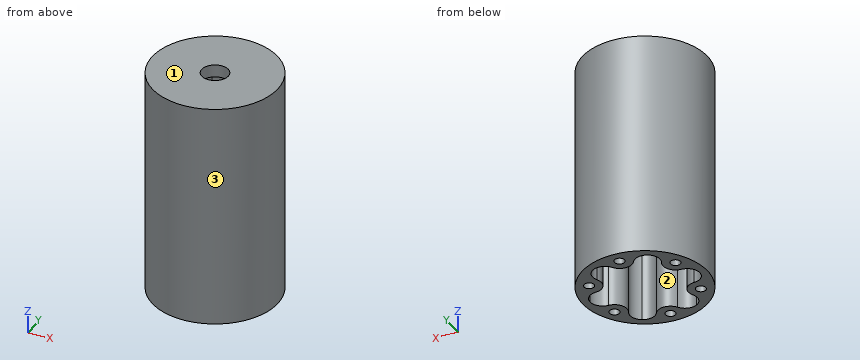
Autodesk Inventor part; units mm, degrees
ref_plane "YZ Plane" through (0, 0, 0) normal (1, 0, 0) x (0, 1, 0)
ref_plane "XZ Plane" through (0, 0, 0) normal (0, 1, 0) x (-1, 0, 0)
ref_plane "XY Plane" through (0, 0, 0) normal (0, 0, 1) x (1, 0, 0)
sketch "Sketch1" plane through (0, 0, 0) normal (0, 0, 1) x (1, 0, 0)
  circle A0 centre (0, 0) radius 15.875
  circle A1 centre (0, 0) radius 13.97
  dimension "d0" = 31.75
  dimension "d1" = 27.94
extrude "Extrusion1" add sketch "Sketch1" along normal blind 57.15
sketch "Sketch2" plane through (0, 0, 0) normal (0, 0, -1) x (-1, 0, 0)
  line L0 (0, 0) -> (0, 12.7)
  circle A0 centre (0, 12.7) radius 1.27
  circle A1 centre (0, 12.7) radius 3.175
  circle A2 centre (-10.9985, 6.35) radius 3.175
  circle A3 centre (-10.9985, 6.35) radius 1.27
  circle A4 centre (-10.9985, -6.35) radius 3.175
  circle A5 centre (-10.9985, -6.35) radius 1.27
  circle A6 centre (0, -12.7) radius 3.175
  circle A7 centre (0, -12.7) radius 1.27
  circle A8 centre (10.9985, -6.35) radius 3.175
  circle A9 centre (10.9985, -6.35) radius 1.27
  circle A10 centre (10.9985, 6.35) radius 3.175
  circle A11 centre (10.9985, 6.35) radius 1.27
  dimension "d4" = 12.7
  dimension "d5" = 2.54
  dimension "d6" = 6.35
  dimension "d9" = 360
extrude "Extrusion2" add sketch "Sketch2" against normal up to surface (57.15 mm away) contours A0 | A1 | A2 | A3 | A4 | A5 | A6 | A7 | A8 | A9 | A10 | A11
extrude "Extrusion3" cut sketch "Sketch2" against normal blind 12.7 contours A0 | A3 | A5 | A7 | A9 | A11
sketch "Sketch3" plane through (0, 0, 57.15) normal (0, 0, 1) x (1, 0, 0)
  circle A0 centre (0, 0) radius 3.3655
  circle A1 centre (0, 0) radius 13.97
  dimension "d15" = 6.731
extrude "Extrusion4" add sketch "Sketch3" against normal blind 3.175
fillet "Fillet1" radius 3.175 12 edges at (-3.0337, 13.6366, 26.9875) (3.0337, 13.6366, 26.9875) (13.3265, 4.191, 26.9875) (10.2928, 9.4456, 26.9875) (13.3265, -4.191, 26.9875) (10.2928, -9.4456, 26.9875) (3.0337, -13.6366, 26.9875) (-3.0337, -13.6366, 26.9875) (-10.2928, -9.4456, 26.9875) (-13.3265, -4.191, 26.9875) (-13.3265, 4.191, 26.9875) (-10.2928, 9.4456, 26.9875)
properties part number "FixedCylinderWireStorage" material "ABS Plastic"
Could you check a few things on this model? Use its own coordinates, in mm. Face numbers are marked on the shaded views. Round coordinates to 2 decimals unless told otherwise and drop trailing zeros. Put each result on its own line as item: value.
Q1. Please list where these lines run through material, in increasing order: line 1 (X direction, y = 11, z = 50); line 2 (Z direction, x = -5.5, y = 10.5) (3 decimals); line 3 (Y direction, x = -5, z = 8.5). Write a range as from..to.
Checks:
line 1: -11.45..-8.11, -2.68..2.68, 8.11..11.45
line 2: 53.975..57.15
line 3: -15.07..-12.5, 12.5..15.07
Q2. Thinking about a two-plate mould opening in Y: for the marked faces 1, 2 and 3, which applies, pulls with the +Y half, pulls with the -Y half, needs draft (parallel to the pull), parting line crosses it, or undercut?
Checks:
face 1: needs draft
face 2: undercut
face 3: parting line crosses it
Q3. For pin 1 Ø6 at (x, z) = (10.5, 11) entering from +Y; pin 2 Ø4 at (x, y) = (0, 0) entering from -Z; pin 3 Ø0.8 at (x, y) = (11.5, -6.5) entering from -Z; pin 4 Ø6 at (x, z) = (8, 17) entering from +Y, each with a flat end and sliding along its axis, tell me the tip position at first contact or that it passes through.
Checks:
pin 1: y = 13.99
pin 2: through
pin 3: z = 12.7
pin 4: y = 15.07
